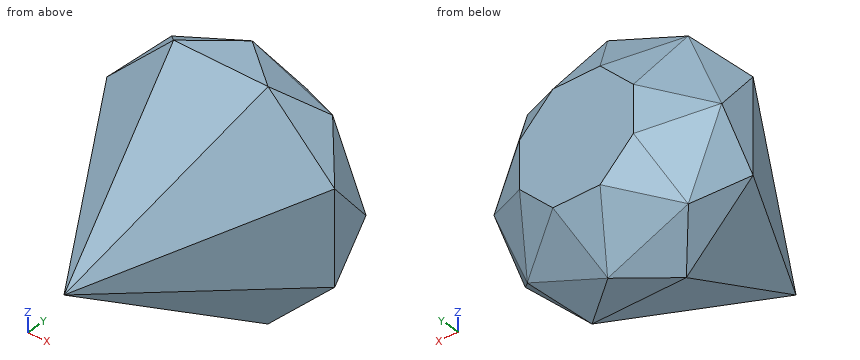
from build123d import *

# Parameters (mm, degrees)
BOSS_EXTRUDE1_DEPTH = 70
CUT_EXTRUDE1_DEPTH  = 13.426406871
CIRPATTERN1_COUNT   = 8
CUT_EXTRUDE2_DEPTH  = 40.196888946
CIRPATTERN2_COUNT   = 8


with BuildPart() as part:
    # Sketch1 → Boss-Extrude1 (new body)
    with BuildSketch(Plane(origin=(0, 0, 0), x_dir=(1, 0, 0), z_dir=(0, 1, 0))):
        Polygon((0, 0), (-12.426406871, 30), (12.426406871, 30), align=None)
    boss_extrude1 = extrude(amount=BOSS_EXTRUDE1_DEPTH)

    # Sketch2 → Cut-Extrude1 (cut, symmetric)
    with BuildSketch(Plane(origin=(0, 0, 0), x_dir=(0, 0, -1), z_dir=(1, 0, 0))):
        Polygon((15, 70), (30, 60), (30, 70), align=None)
        Polygon((30, 50), (0, 0), (30, 0), align=None)
    cut_extrude1 = extrude(amount=CUT_EXTRUDE1_DEPTH, both=True, mode=Mode.SUBTRACT)

    # CirPattern1: Boss-Extrude1, Cut-Extrude1 ×8 about axis
    cirpattern1_axis = Axis((0, 0, 0), (0, 1, 0))
    for i in range(1, CIRPATTERN1_COUNT):
        add(boss_extrude1.rotate(cirpattern1_axis, i * 360 / CIRPATTERN1_COUNT))
        add(cut_extrude1.rotate(cirpattern1_axis, i * 360 / CIRPATTERN1_COUNT), mode=Mode.SUBTRACT)

    # Sketch3 → Cut-Extrude2 (cut, symmetric)
    with BuildSketch(Plane(origin=(0, 0, 0), x_dir=(0, 1, 0), z_dir=(0.923879533, 0, -0.382683432))):
        Polygon((70, 32.471766009), (70, 16.235883004), (60, 27.7), (50, 32.471766009), align=None)
    cut_extrude2 = extrude(amount=CUT_EXTRUDE2_DEPTH, both=True, mode=Mode.SUBTRACT)

    # CirPattern2: Cut-Extrude2 ×8 about axis
    cirpattern2_axis = Axis((0, 0, 0), (0, 1, 0))
    for i in range(1, CIRPATTERN2_COUNT):
        add(cut_extrude2.rotate(cirpattern2_axis, i * 360 / CIRPATTERN2_COUNT), mode=Mode.SUBTRACT)


solid = part.part
Work out the finished part from the listing and answer in its coordinate system (mm). Give positions to 0.01 mm unless a question says otherwise; leave off trailing zeros. Write each loop counter-clockwise with the first axis right and the second up, starting at its lowest first coordinate (ties: lowest second). Pieces come first, ordered by that corner, then holes. Notation, with made-up numbers: (72, 65) - (87, 65) arc R11 ccw to (87, 70) - close; hole circle Ø6 at (39.25, 28.25). An arc over 180 degrees is marked (long way). One line per item, written item: value. Start each with the question number.
1. Given pin 1 (6 mm diameter, centred on y = 7.5, z = -4, fed in from -X); pin 2 (1 mm diameter, centred on y = 46.5, z = 0, fed in from -X); pin 3 (4 mm diameter, centred on y = 43, z = 15, fed in from +X), each flat-ended and moving along its own axis, determine where each tip first touches the part or whether it passes through.
2. Find section B-B (y = 63.5). Write down the section's boundary in (x, z), then the cut area to 3 significant figures.
3. Find section A-A (z = 4.5). Write down the section's boundary in (x, y).
4. Find section C-C (x = -26). Write down the section's boundary in (y, z).
5. Consider probe 1 along Z at (x, y) = (-7.5, 17); probe 2 along Y at (x, z) = (-8, 22.5); probe 3 along Z at (x, y) = (-26, 50.5). Determine where each line is inside the solid, lowest interval first.
6. Find section D-D (z = 25). Write down the section's boundary in (x, y).
Geometry results:
1. pin 1: x = -6.06
1. pin 2: x = -28.2
1. pin 3: x = 24.11
2. outline: (-24.75, -2.15) - (-19.02, -15.98) - (-15.98, -19.02) - (-2.15, -24.75) - (2.15, -24.75) - (15.98, -19.02) - (19.02, -15.98) - (24.75, -2.15) - (24.75, 2.15) - (19.02, 15.98) - (15.98, 19.02) - (2.15, 24.75) - (-2.15, 24.75) - (-15.98, 19.02) - (-19.02, 15.98) - (-24.75, 2.15) - close
2. area: 1,840 mm2
3. outline: (-30, 50) - (-10.86, 18.11) - (-1.86, 7.5) - (1.86, 7.5) - (10.86, 18.11) - (30, 50) - (30, 56.36) - (28.12, 60) - (19.11, 67.26) - (15, 70) - (-15, 70) - (-19.11, 67.26) - (-28.12, 60) - (-30, 56.36) - close
4. outline: (43.33, -10.77) - (50, -16.43) - (54.54, -16.43) - (60, -9.61) - (62.67, -1.63) - (62.67, 1.63) - (60, 9.61) - (54.54, 16.43) - (50, 16.43) - (43.33, 10.77) - close
5. probe 1: -6.92 to 6.92
5. probe 2: 37.5 to 63.36
5. probe 3: -16.43 to 16.43
6. outline: (-17.43, 50) - (-10.36, 41.67) - (10.36, 41.67) - (17.43, 50) - (17.43, 55.67) - (12.03, 60) - (2.04, 63.33) - (-2.04, 63.33) - (-12.03, 60) - (-17.43, 55.67) - close
